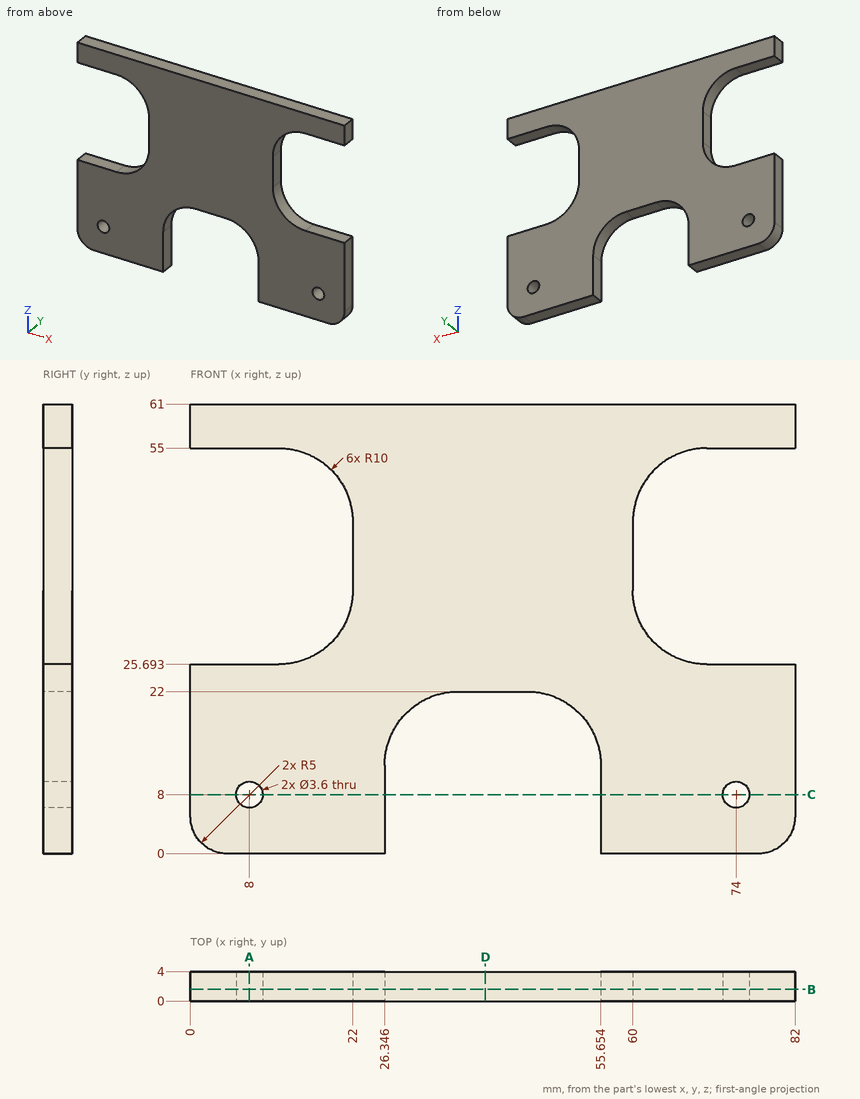
The drawing under review shows one solid part. Ordinate dimensions are in mm from its lowest x, y, z. Give positions to 0.01 mm unless a question says otherwise; leave off trailing zeros. Write each loop counter-clockwise with the first axis right and the second up, starting at its lowest first coordinate (ties: lowest second). Pieces come first, ordered by that corner, then holes. Notation, with made-up numbers: M 6,60 L 49,60 A32 ccw 49,92 Z; hole C 77,29.5 d8. An arc over 180 degrees is marked long. Write each question's results on one line, items separated by ' | '. Start each with the question number.
1. We need section A-A (x = 8). Write out the cut boundary in (y, z), and give its area (3 significant figures).
2. We need section B-B (y = 1.6). Write out the cut boundary in (x, z).
3. We need section C-C (z = 8). Write out the cut boundary in (x, y), and give its area (3 significant figures).
4. Insertion check: pin 1 Ø1.2 at (x, y) = (41, 1) entering from -Z; pin 2 Ø2 at (x, y) = (51.5, 2.5) entering from -Z; pin 3 Ø1.5 at (y, z) = (3.5, 31.5) entering from +X. Each pin has a flat end and moves straight along its axis. Give the tip position at first contact, or say it passes through.
5. We need section D-D (x = 40). Write out the cut boundary in (y, z).
6. For probe 1 along X at (y, z) = (2.55, 8); probe 2 along X at (y, z) = (3.75, 11); probe 3 along Z at (x, y) = (11.5, 1.9), list the stretches that pass through material, from the lowest coordinate up. Write a range as [from, to].
Results found:
1) outline: M 0,0 L 4,0 L 4,6.2 L 0,6.2 Z; M 0,9.8 L 4,9.8 L 4,25.69 L 0,25.69 Z; M 0,55 L 4,55 L 4,61 L 0,61 Z | area: 112 mm^2
2) outline: M 0,5 A5 ccw 5,0 L 26.35,0 L 26.35,12 A10 cw 36.35,22 L 45.65,22 A10 cw 55.65,12 L 55.65,0 L 77,0 A5 ccw 82,5 L 82,25.69 L 70,25.69 A10 cw 60,35.69 L 60,45 A10 cw 70,55 L 82,55 L 82,61 L 0,61 L 0,55 L 12,55 A10 cw 22,45 L 22,35.69 A10 cw 12,25.69 L 0,25.69 Z; hole C 8,8 d3.6; hole C 74,8 d3.6
3) outline: M 0,0 L 6.2,0 L 6.2,4 L 0,4 Z; M 9.8,0 L 26.35,0 L 26.35,4 L 9.8,4 Z; M 55.65,0 L 72.2,0 L 72.2,4 L 55.65,4 Z; M 75.8,0 L 82,0 L 82,4 L 75.8,4 Z | area: 182 mm^2
4) pin 1: stops at z = 22 | pin 2: stops at z = 19.29 | pin 3: stops at x = 61.31
5) outline: M 0,22 L 4,22 L 4,61 L 0,61 Z
6) probe 1: x = [0, 6.2], [9.8, 26.35], [55.65, 72.2], [75.8, 82] | probe 2: x = [0, 26.35], [55.65, 82] | probe 3: z = [0, 25.69], [55, 61]
